```python
from build123d import *

# Parameters (mm, degrees)
SKETCH1_W               = 38
SKETCH1_H               = 52
EXTRUDE1_DEPTH          = 15
SKETCH3_R               = 3.175
CUT_EXTRUDE2_DEPTH      = 18
SKETCH5_W               = 12
SKETCH5_H               = 15
CUT_EXTRUDE4_DEPTH      = 4
F_1_4_CLEARANCE_HOLE1_D = 6.5278
CUT_EXTRUDE5_REACH      = 17
SKETCH12_R              = 0.508


with BuildPart() as part:
    # Sketch1 → Extrude1 (new body)
    with BuildSketch(Plane.XY):
        with Locations((0, 26)):
            Rectangle(SKETCH1_W, SKETCH1_H)
    extrude(amount=EXTRUDE1_DEPTH)

    # Sketch3 → Cut-Extrude2 (cut)
    with BuildSketch(Plane(origin=(0, 52, 0), x_dir=(-1, 0, 0), z_dir=(0, 1, 0))):
        with Locations(Location((12.5, 7.5, 0), (0, 0, 90))):  # turned: the seam where the file's is
            Circle(SKETCH3_R)
        with Locations(Location((-12.5, 7.5, 0), (0, 0, 270))):  # turned: the seam where the file's is
            Circle(SKETCH3_R)
    extrude(amount=-CUT_EXTRUDE2_DEPTH, mode=Mode.SUBTRACT)

    # Sketch5 → Cut-Extrude4 (cut)
    with BuildSketch(Plane(origin=(0, 52, 0), x_dir=(-1, 0, 0), z_dir=(0, 1, 0))):
        with Locations((0, 7.5)):
            Rectangle(SKETCH5_W, SKETCH5_H)
    extrude(amount=-CUT_EXTRUDE4_DEPTH, mode=Mode.SUBTRACT)

    # 1/4 Clearance Hole1 (through all)
    with Locations(Plane(origin=(0, 48, 0), x_dir=(-1, 0, 0), z_dir=(0, 1, 0))):
        with Locations((0, 7.5)):
            Hole(F_1_4_CLEARANCE_HOLE1_D / 2)

    # Sketch12 → Cut-Extrude5 (cut, up to next)
    with BuildSketch(Plane.XY.offset(15), mode=Mode.PRIVATE) as cut_extrude5_sk1:
        with Locations((-12.5, 39.3)):
            Circle(SKETCH12_R)
    cut_extrude5_tool1 = extrude(cut_extrude5_sk1.sketch, amount=-CUT_EXTRUDE5_REACH, mode=Mode.PRIVATE) & part.part
    add(cut_extrude5_tool1.solids().sort_by_distance((-12.5, 39.3, 15))[0], mode=Mode.SUBTRACT)
    # Sketch12 → Cut-Extrude5 (cut, up to next)
    with BuildSketch(Plane.XY.offset(15), mode=Mode.PRIVATE) as cut_extrude5_sk2:
        with Locations((12.5, 39.3)):
            Circle(SKETCH12_R)
    cut_extrude5_tool2 = extrude(cut_extrude5_sk2.sketch, amount=-CUT_EXTRUDE5_REACH, mode=Mode.PRIVATE) & part.part
    add(cut_extrude5_tool2.solids().sort_by_distance((12.5, 39.3, 15))[0], mode=Mode.SUBTRACT)


solid = part.part
```
Input: part model. Units: mm. Frame: model coordinates. A direction names the side the tool comes from. Coordinates: 2 decimals unless noted, no trailing zeros. Order: outer loops, then holes, each group sorted by start corner. A loop starts at its lowest first (then second) coordinate and runs counter-clockwise, first axis right, second up. Notation, with made-up numbers: (-37.5, -26.75) - (-30.5, -26.75) arc R13 ccw to (-30.5, -6.75) - close; hole circle Ø1 at (71.25, -37.5). An arc over 180 degrees is marked (long way). Put each result on its own line as item: value.
1. Line query: line 1 along X through (y, z) = (39.3, 13.2); line 2 along X through (y, z) = (42, 7.75); line 3 along Y through (x, z) = (5, 3). Output: solid intervals per line, ascending.
Report:
line 1: x = -19 to -13.01, -11.99 to 11.99, 13.01 to 19
line 2: x = -19 to -15.67, -9.33 to -3.25, 3.25 to 9.33, 15.67 to 19
line 3: y = 0 to 48
2. Cut plane C-C on y = 43. Return the cut outline in (x, z) (3 decimals).
Report:
outline: (-19, 0) - (19, 0) - (19, 15) - (-19, 15) - close; hole circle Ø6.35 at (-12.5, 7.5); hole circle Ø6.528 at (0, 7.5); hole circle Ø6.35 at (12.5, 7.5)
3. Reachability of faces 1 (the face through (-12.6, 39.8, 12.8)), 2 (the face through (12, 34, 8)), 3 (the face through (0, 48, 11)) from +Z, -Z, +X, -X, +Y, -Y: full face, straight path, thin tool, end or side. Return the list, or none.
Report:
face 1: +Z
face 2: +Y
face 3: +Z, -Z, +Y
4. Cut plane B-B on z = 2. Return the cut outline in (x, y).
Report:
outline: (-19, 0) - (19, 0) - (19, 52) - (6, 52) - (6, 48) - (-6, 48) - (-6, 52) - (-19, 52) - close
5. Cut plane D-D on y = 21. Return the cut outline in (x, z).
Report:
outline: (-19, 0) - (19, 0) - (19, 15) - (-19, 15) - close; hole circle Ø6.53 at (0, 7.5)
6. Cut plane A-A on x = 0. Return the cut outline in (y, z), then the cut area to 3 significant figures.
Report:
outline: (0, 0) - (48, 0) - (48, 4.24) - (0, 4.24) - close; (0, 10.76) - (48, 10.76) - (48, 15) - (0, 15) - close
area: 407 mm2
7. Contact query for a flat-ended pin moving along its axis: pin 1 Ø3.5 at (x, z) = (-2.5, 4) entering from +Y. Output: stop coordinate, or through.
Report:
pin 1: stops at y = 48
8. Draft query along X for faces 4 (the face through (12.4, 39.8, 12.8)), 5 (the face through (19, 26, 7)), 6 (the face through (-19, 26, 7)), 7 (the face through (-13, 52, 11)). Return one class per face: pulls with the +X half, pulls with the -X half, needs draft (parallel to the pull), parting line crosses it, or undercut.
Report:
face 4: undercut
face 5: pulls with the +X half
face 6: pulls with the -X half
face 7: needs draft
